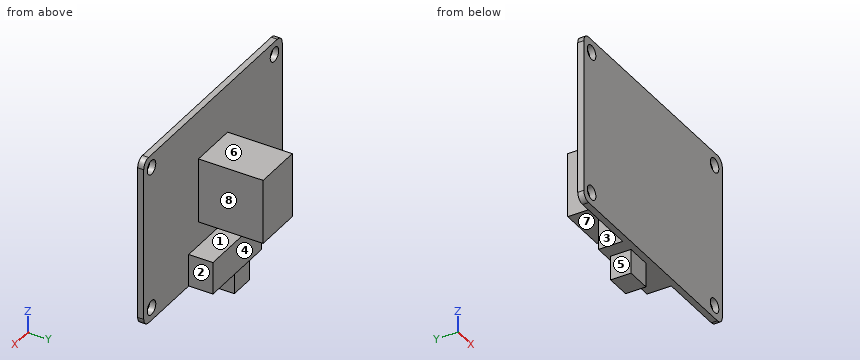
```python
from build123d import *

# Parameters (mm, degrees)
SKETCH1_W           = 57
SKETCH1_H           = 42
BOSS_EXTRUDE1_DEPTH = 1.5
SKETCH2_R           = 1.75
CUT_EXTRUDE1_DEPTH  = 10
SKETCH3_W           = 12
SKETCH3_H           = 16
SKETCH3_W_2         = 20
SKETCH3_H_2         = 8
BOSS_EXTRUDE2_DEPTH = 6
SKETCH4_W           = 6.209741393
SKETCH4_H           = 5.053024859
BOSS_EXTRUDE3_DEPTH = 6
FILLET3_R           = 2
SKETCH7_W           = 12
SKETCH7_H           = 16
BOSS_EXTRUDE6_DEPTH = 10


with BuildPart() as part:
    # Sketch1 → Boss-Extrude1 (new body)
    with BuildSketch(Plane(origin=(0, 0, 0), x_dir=(1, 0, 0), z_dir=(0, 1, 0))):
        Rectangle(SKETCH1_W, SKETCH1_H)
    extrude(amount=BOSS_EXTRUDE1_DEPTH)

    # Sketch2 → Cut-Extrude1 (cut)
    with BuildSketch(Plane(origin=(0, 1.5, 0), x_dir=(1, 0, 0), z_dir=(0, 1, 0))):
        with Locations(Location((-25.3, 17.8, 0), (0, 0, 270))):
            Circle(SKETCH2_R)
        with Locations(Location((-25.3, -17.8, 0), (0, 0, 270))):
            Circle(SKETCH2_R)
        with Locations(Location((25.3, -17.8, 0), (0, 0, 270))):
            Circle(SKETCH2_R)
        with Locations(Location((25.3, 17.8, 0), (0, 0, 270))):
            Circle(SKETCH2_R)
    extrude(amount=-CUT_EXTRUDE1_DEPTH, mode=Mode.SUBTRACT)

    # Sketch3 → Boss-Extrude2 (add)
    with BuildSketch(Plane(origin=(0, 1.5, 0), x_dir=(1, 0, 0), z_dir=(0, 1, 0))):
        with Locations((0, -1)):
            Rectangle(SKETCH3_W, SKETCH3_H)
        with Locations((0, 17)):
            Rectangle(SKETCH3_W_2, SKETCH3_H_2)
    extrude(amount=BOSS_EXTRUDE2_DEPTH)

    # Sketch4 → Boss-Extrude3 (add)
    with BuildSketch(Plane(origin=(0, 0, -21), x_dir=(-1, 0, 0), z_dir=(0, 0, -1))):
        with Locations((3.348389967, 4.115278906)):
            Rectangle(SKETCH4_W, SKETCH4_H)
    extrude(amount=BOSS_EXTRUDE3_DEPTH)

    # Fillet3
    fillet3_edges = [part.edges().sort_by_distance(p)[0] for p in [
        (28.5, 0.75, 21),
        (-28.5, 0.75, 21),
        (-28.5, 0.75, -21),
        (28.5, 0.75, -21),
    ]]
    fillet(fillet3_edges, radius=FILLET3_R)

    # Sketch7 → Boss-Extrude6 (add)
    with BuildSketch(Plane(origin=(0, 7.5, 0), x_dir=(1, 0, 0), z_dir=(0, 1, 0))):
        with Locations((0, -1)):
            Rectangle(SKETCH7_W, SKETCH7_H)
    extrude(amount=BOSS_EXTRUDE6_DEPTH)


solid = part.part
```
Check sheet for the modelled part. Datum: model origin and axes. Units: mm. Face numbers are marked on the shaded views. A direction names the side the tool comes from. Give positions to 0.01 mm unless a question says otherwise; leave off trailing zeros. Write each loop counter-clockwise with the first axis right and the second up, starting at its lowest first coordinate (ties: lowest second). Pieces come first, ordered by that corner, then holes. Notation, with made-up numbers: (-5.75, 31.5) -> (21.25, 31.5) arc R12 ccw to (21.25, 46.5) -> close; hole circle Ø3 at (-7, -17). An arc over 180 degrees is marked (long way). Use CSV: the item, a comma, the result in double quotes. Start each with the question number.
Q1. Tool access check on the marked faces 1, 2, 3, 4 and 5. Record the directions out of +Z, -Z, +X, -X, +Y, -Y that give a thin tool (end or side, any length) a straight path to the whole face; none if there is none.
Q2. Cross-section at D-D on z = -4.5. Enter the section's corners in (x, y), and give its area (4 significant figures).
Q3. Cross-section at A-A on y = 3.25. Enter the section's corners in (x, z), and give its area (3 significant figures).
Q4. Depth check by flat-ended pin: P1, Ø1.8, axis at y = 4, z = -18, coming from the +X side; P2, Ø1.5, axis at y = 4.5, z = -25, coming from the +X side; P3, Ø3, axis at x = -25.3, z = -17.8, coming from the -Y side (3 decimals); P4, Ø5.5, axis at x = -25.3, z = 17.8, coming from the +Y side. Enter the tip coordinate at first touch or a pass-through.
Q5. Scan lines: line 1 along X through (y, z) = (1.15, 17.8); line 2 along Z through (x, y) = (3.5, 6.75); line 3 along Z through (x, y) = (-1, 10). Record each from-to range of solid material in increasing order.
Q6. Cross-section at B-B on z = 17.8. Enter the section's corners in (x, y), and give its area (3 significant figures).
Q7. Cross-section at C-C on x = -25.3. Enter the section's corners in (y, z).
Q8. Release check for a two-part mould opening along Z. For the marked faces 6, 7 and 8 record: +Z half, -Z half, draft (parallel to the pull), parting line (faces both ways), or undercut.
Working result:
1,face 1,"+X, -X, +Y"
1,face 2,"+Z, -Z, +X, +Y"
1,face 3,"+Z, -Z, -X, +Y"
1,face 4,"-Z, +X, -X, +Y"
1,face 5,"-Z, -X, +Y, -Y"
2,outline,"(-28.5, 0) -> (28.5, 0) -> (28.5, 1.5) -> (6, 1.5) -> (6, 17.5) -> (-6, 17.5) -> (-6, 1.5) -> (-28.5, 1.5) -> close"
2,area,"277.5 mm^2"
3,outline,"(-10, -21) -> (-6.45, -21) -> (-6.45, -27) -> (-0.24, -27) -> (-0.24, -21) -> (10, -21) -> (10, -13) -> (-10, -13) -> close; (-6, -7) -> (6, -7) -> (6, 9) -> (-6, 9) -> close"
3,area,"389 mm^2"
4,P1,"stops at x = 10"
4,P2,"stops at x = -0.24"
4,P3,"passes through"
4,P4,"stops at y = 1.5"
5,line 1,"x = -28.5 to -27.05, -23.55 to 23.55, 27.05 to 28.5"
5,line 2,"z = -21 to -13, -7 to 9"
5,line 3,"z = -7 to 9"
6,outline,"(-28.5, 0) -> (-27.05, 0) -> (-27.05, 1.5) -> (-28.5, 1.5) -> close; (-23.55, 0) -> (23.55, 0) -> (23.55, 1.5) -> (-23.55, 1.5) -> close; (27.05, 0) -> (28.5, 0) -> (28.5, 1.5) -> (27.05, 1.5) -> close"
6,area,"75.0 mm^2"
7,outline,"(0, -21) -> (1.5, -21) -> (1.5, -19.55) -> (0, -19.55) -> close; (0, -16.05) -> (1.5, -16.05) -> (1.5, 16.05) -> (0, 16.05) -> close; (0, 19.55) -> (1.5, 19.55) -> (1.5, 21) -> (0, 21) -> close"
8,face 6,"+Z half"
8,face 7,"undercut"
8,face 8,"draft"
